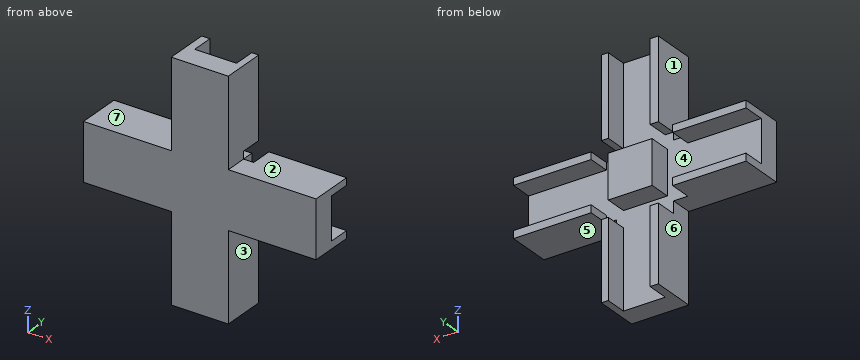
```python
from build123d import *

# Parameters (mm, degrees)
BOSS_EXTRUDE1_DEPTH = 10
SKETCH3_W           = 20
SKETCH3_H           = 20
BOSS_EXTRUDE2_DEPTH = 10
SKETCH4_W           = 33.498835794
SKETCH4_H           = 3.393870965
SKETCH4_H_2         = 3.249417897
SKETCH4_W_2         = 3.755003636
SKETCH4_H_3         = 36.60457676
SKETCH4_W_3         = 3.177191363
SKETCH4_W_4         = 35.376725681
SKETCH4_H_4         = 35.593405283
SKETCH4_H_5         = 34.582233806
BOSS_EXTRUDE3_DEPTH = 10


with BuildPart() as part:
    # Sketch1 → Boss-Extrude1 (new body)
    with BuildSketch(Plane(origin=(0, 0, 0), x_dir=(1, 0, 0), z_dir=(0, 1, 0))):
        Polygon((-12.830188679, 53), (-12.830188679, 13), (-52.830188679, 13), (-52.830188679, -13), (-12.830188679, -13), (-12.830188679, -53), (13.169811321, -53), (13.169811321, -13), (53.169811321, -13), (53.169811321, 13), (13.169811321, 13), (13.169811321, 53), align=None)
    extrude(amount=-BOSS_EXTRUDE1_DEPTH)

    # Sketch3 → Boss-Extrude2 (add)
    with BuildSketch(Plane(origin=(0, 0, 0), x_dir=(1, 0, 0), z_dir=(0, 1, 0))):
        Rectangle(SKETCH3_W, SKETCH3_H)
    extrude(amount=BOSS_EXTRUDE2_DEPTH)

    # Sketch4 → Boss-Extrude3 (add)
    with BuildSketch(Plane(origin=(0, 0, 0), x_dir=(1, 0, 0), z_dir=(0, 1, 0))):
        with Locations((-36.080770782, 11.303064518)):
            Rectangle(SKETCH4_W, SKETCH4_H)
        with Locations((-36.080770782, -11.375291051)):
            Rectangle(SKETCH4_W, SKETCH4_H_2)
        with Locations((-10.952686861, -34.69771162)):
            Rectangle(SKETCH4_W_2, SKETCH4_H_3)
        with Locations((11.58121564, -34.69771162)):
            Rectangle(SKETCH4_W_3, SKETCH4_H_3)
        with Locations((35.481448481, -11.375291051)):
            Rectangle(SKETCH4_W_4, SKETCH4_H_2)
        with Locations((35.481448481, 11.303064518)):
            Rectangle(SKETCH4_W_4, SKETCH4_H)
        with Locations((11.58121564, 35.203297359)):
            Rectangle(SKETCH4_W_3, SKETCH4_H_4)
        with Locations((-10.952686861, 35.708883097)):
            Rectangle(SKETCH4_W_2, SKETCH4_H_5)
    extrude(amount=BOSS_EXTRUDE3_DEPTH)


solid = part.part
```
Check sheet for the modelled part. Datum: model origin and axes. Units: mm. Face numbers are marked on the shaded views. A direction names the side the tool comes from. Round coordinates to 2 decimals unless told otherwise and drop trailing zeros. Order: outer loops, then holes, each group sorted by start corner. A loop starts at its lowest first (then second) coordinate and runs counter-clockwise, first axis right, second up. Notation, with made-up numbers: (-31, -31.5) -> (-11, -31.5) arc R6 ccw to (-11, -22.5) -> close; hole circle Ø11 at (-10, -25). An arc over 180 degrees is marked (long way). One line per item, written item: value. Start each with the question number.
Q1. Cross-section at C-C (x = -6). Record the boundary of the cut face in (y, z).
Q2. Set-up check for the marked faces 5, 6 and 7: record each of +Z, -Z, +X, -X, +Y, -Y from which the full face is reachable in a straight line by a thin tool's end or side.
Q3. Mould release check, pull along X, two halves, no side actions. Record for the marked faces 1, 2, 3 and 4: pulls with the +X half, pulls with the -X half, needs draft (parallel to the pull), parting line crosses it, or undercut.
Q4. Gauge pin test, flat ends, axial feed: pin 1 Ø6 at (x, y) = (36.5, 2.5) entering from -Z; pin 2 Ø3 at (x, z) = (-15.5, 32.5) entering from +Y; pin 3 Ø8 at (x, y) = (41.5, 4) entering from +Z; pin 4 Ø3 at (y, z) = (4.5, 21.5) entering from +X. Record the tip position at first contact, or that the pin passes through.
Q5. Thickness scan on line 1 (Z direction, x = 31, y = 2.5); line 2 (X direction, y = 7, z = 22); line 3 (Y direction, x = -3.5, z = -47.5). Record the ranges inside material, lowest first.
Q6. Cross-section at B-B (y = 1.5). Give the number of separate pieces and of enclosed holes in the cut face, and give its area (3 significant figures).
Q7. Cross-section at A-A (z = 27). Record the boundary of the cut face in (x, y).
Q8. Cross-section at D-D (z = 14.5). Record the boundary of the cut face in (x, y).
Completed:
1. outline: (-10, -53) -> (0, -53) -> (0, -10) -> (10, -10) -> (10, 10) -> (0, 10) -> (0, 53) -> (-10, 53) -> close
2. face 5: -Z, +X, +Y, -Y
2. face 6: -Z, -X, +Y, -Y
2. face 7: +Z, -X, +Y, -Y
3. face 1: pulls with the -X half
3. face 2: needs draft
3. face 3: pulls with the +X half
3. face 4: undercut
4. pin 1: stops at z = -13
4. pin 2: passes through
4. pin 3: stops at z = 13
4. pin 4: stops at x = 13.17
5. line 1: z = -13 to -9.61, 9.75 to 13
5. line 2: x = -12.83 to -9.08, 9.99 to 13.17
5. line 3: y = -10 to 0
6. separate pieces: 9
6. enclosed holes: 0
6. area: 1,350 mm²
7. outline: (-12.83, -10) -> (13.17, -10) -> (13.17, 10) -> (9.99, 10) -> (9.99, 0) -> (-9.08, 0) -> (-9.08, 10) -> (-12.83, 10) -> close
8. outline: (-12.83, -10) -> (13.17, -10) -> (13.17, 0) -> (-12.83, 0) -> close
